Read the model definition and answer for the solid it produces. Units are mm, in the model's axes. Face numbers are marked on the shaded views. A direction names the side the tool comes from. Give positions to 0.01 mm unless a question says otherwise; leave off trailing zeros. Write each loop counter-clockwise with the first axis right and the second up, starting at its lowest first coordinate (ties: lowest second). Pieces come first, ordered by that corner, then holes. Notation, with made-up numbers: (-14.5, 25) -> (31.5, 25) arc R10 cw to (31.5, 42) -> close; hole circle Ø10 at (-33.75, 67.25). An arc over 180 degrees is marked (long way). Use a Markdown table: item, result.
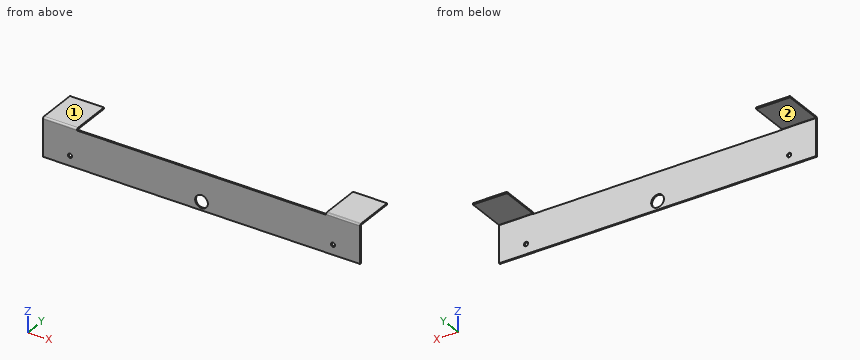
from build123d import *

# Parameters (mm, degrees)
SKETCH18_W                   = 711.2
SKETCH18_H                   = 3.175
BASE_FLANGE1_DEPTH           = 174.625
SKETCH23_W                   = 215.9
SKETCH23_H                   = 88.9
CUT_EXTRUDE1_DEPTH           = 630.633777431
SKETCH24_W                   = 127
SKETCH24_H                   = 34.925
CUT_EXTRUDE2_DEPTH           = 630.633777431
SKETCH25_W                   = 215.9
SKETCH25_H                   = 88.9
CUT_EXTRUDE3_DEPTH           = 630.633777431
SKETCH32_W                   = 558.8
SKETCH32_H                   = 92.075
CUT_EXTRUDE6_DEPTH           = 630.633777431
SKETCHED_START               = -106.274614162
SKETCHED_BEND1_OUTLINE_W     = 3.175
SKETCHED_BEND1_OUTLINE_H     = 88.9
SKETCHED_BEND1_OUTLINE_H_2   = 82.55
SKETCHED_BEND1_DEPTH         = 635
SKETCHED_START_2             = 528.725385838
SKETCHED_BEND1_2_DEPTH       = 76.2
SKETCHED_BEND1_3_OUTLINE_W   = 82.55
SKETCHED_BEND1_3_OUTLINE_H   = 3.175
SKETCHED_BEND1_3_DEPTH       = 711.2
SKETCHED_BEND1_4_OUTLINE_W   = 0.997512257
SKETCHED_BEND1_4_OUTLINE_H   = 3.175
SKETCHED_BEND1_4_OUTLINE_W_2 = 87.902487743
SKETCHED_BEND1_4_DEPTH       = 76.2
SKETCHED_BEND1_5_DEPTH       = 76.2
SKETCHED_BEND2_DEPTH         = 711.2
SKETCHED_BEND2_2_OUTLINE_W   = 3.175
SKETCHED_BEND2_2_OUTLINE_H   = 82.55
SKETCHED_BEND2_2_DEPTH       = 711.2
SKETCHED_BEND2_3_DEPTH       = 76.2
SKETCHED_BEND2_4_DEPTH       = 76.2
SKETCH35_R                   = 14.2875
SKETCH35_R_2                 = 4.7625
CUT_EXTRUDE7_DEPTH           = 619.781329454


# Read off the part's stored shape, not the designer's step: Sketched Bend1, Sketched Bend2
# Sheet-metal steps are written as plain solids
with BuildPart() as part:
    # Sketch18 → Base-Flange1 (new body)
    with BuildSketch(Plane.XY):
        with Locations((249.325385838, -1.5875)):
            Rectangle(SKETCH18_W, SKETCH18_H)
    extrude(amount=BASE_FLANGE1_DEPTH)

    # Sketch23 → Cut-Extrude1 (cut, through all)
    with BuildSketch(Plane(origin=(0, 0, 0), x_dir=(1, 0, 0), z_dir=(0, 1, 0))):
        with Locations((77.875385838, -44.45)):
            Rectangle(SKETCH23_W, SKETCH23_H)
    extrude(amount=-CUT_EXTRUDE1_DEPTH, mode=Mode.SUBTRACT)

    # Sketch24 → Cut-Extrude2 (cut, through all)
    with BuildSketch(Plane(origin=(0, 0, 0), x_dir=(1, 0, 0), z_dir=(0, 1, 0))):
        with Locations((249.325385838, -17.4625)):
            Rectangle(SKETCH24_W, SKETCH24_H)
    extrude(amount=-CUT_EXTRUDE2_DEPTH, mode=Mode.SUBTRACT)

    # Sketch25 → Cut-Extrude3 (cut, through all)
    with BuildSketch(Plane(origin=(0, 0, 0), x_dir=(1, 0, 0), z_dir=(0, 1, 0))):
        with Locations((420.775385838, -44.45)):
            Rectangle(SKETCH25_W, SKETCH25_H)
    extrude(amount=-CUT_EXTRUDE3_DEPTH, mode=Mode.SUBTRACT)

    # Sketch32 → Cut-Extrude6 (cut, through all)
    with BuildSketch(Plane.XZ.offset(3.175)):
        with Locations((249.325385838, 46.0375)):
            Rectangle(SKETCH32_W, SKETCH32_H)
    extrude(amount=-CUT_EXTRUDE6_DEPTH, mode=Mode.SUBTRACT)

    # Sketched Bend1 outline → Sketched Bend1 (cut)
    with BuildSketch(Plane.YZ.offset(SKETCHED_START)):
        with Locations((-1.5875, 44.45)):
            Rectangle(SKETCHED_BEND1_OUTLINE_W, SKETCHED_BEND1_OUTLINE_H)
        with Locations((-1.5875, 133.35)):
            Rectangle(SKETCHED_BEND1_OUTLINE_W, SKETCHED_BEND1_OUTLINE_H_2)
    extrude(amount=SKETCHED_BEND1_DEPTH, mode=Mode.SUBTRACT)

    # Sketched Bend1 2 outline → Sketched Bend1 2 (cut)
    with BuildSketch(Plane.YZ.offset(SKETCHED_START_2)):
        with BuildLine():
            ThreePointArc((-3.175, 92.005018799), (-0.896479843, 90.655319942), (0, 88.1634))
            Line((0, 88.1634), (0, 174.625))
            Line((0, 174.625), (-3.175, 174.625))
            Line((-3.175, 174.625), (-3.175, 92.005018799))
        make_face()
    extrude(amount=SKETCHED_BEND1_2_DEPTH, mode=Mode.SUBTRACT)



with BuildPart() as body_2:
    # Sketched Bend1 3 outline → Sketched Bend1 3 (new body)
    with BuildSketch(Plane.YZ.offset(SKETCHED_START)):
        with Locations((-45.447512257, 90.4875)):
            Rectangle(SKETCHED_BEND1_3_OUTLINE_W, SKETCHED_BEND1_3_OUTLINE_H)
    extrude(amount=SKETCHED_BEND1_3_DEPTH)


with BuildPart() as part_1:
    add(part.part)

    add(body_2.part)  # Sketched Bend1 4 merges body 2
    # Sketched Bend1 4 outline → Sketched Bend1 4 (add)
    with BuildSketch(Plane.YZ.offset(SKETCHED_START)):
        with Locations((-3.673756128, 90.4875)):
            Rectangle(SKETCHED_BEND1_4_OUTLINE_W, SKETCHED_BEND1_4_OUTLINE_H)
        with Locations((43.951243872, 90.4875)):
            Rectangle(SKETCHED_BEND1_4_OUTLINE_W_2, SKETCHED_BEND1_4_OUTLINE_H)
    extrude(amount=SKETCHED_BEND1_4_DEPTH)

    # Sketched Bend1 5 outline → Sketched Bend1 5 (add)
    with BuildSketch(Plane.YZ.offset(SKETCHED_START_2)):
        with BuildLine():
            Line((-4.172512257, 88.9), (-3.9116, 88.9))
            ThreePointArc((-3.9116, 88.9), (-3.390745145, 88.684254855), (-3.175, 88.1634))
            Line((-3.175, 88.1634), (-3.175, 92.005018799))
            ThreePointArc((-3.175, 92.005018799), (-3.541641581, 92.057465398), (-3.9116, 92.075))
            Line((-3.9116, 92.075), (-4.172512257, 92.075))
            Line((-4.172512257, 92.075), (-4.172512257, 88.9))
        make_face()
    extrude(amount=SKETCHED_BEND1_5_DEPTH)

    # Sketched Bend2 outline → Sketched Bend2 (cut)
    with BuildSketch(Plane.YZ.offset(SKETCHED_START)):
        with BuildLine():
            ThreePointArc((-4.102531056, 88.9), (-2.752832199, 91.178520157), (-0.260912257, 92.075))
            Line((-0.260912257, 92.075), (-86.722512257, 92.075))
            Line((-86.722512257, 92.075), (-86.722512257, 88.9))
            Line((-86.722512257, 88.9), (-4.102531056, 88.9))
        make_face()
        with BuildLine():
            Line((-0.997512257, 5.352487743), (-3.175, 5.352487743))
            Line((-3.175, 5.352487743), (-3.175, 0))
            Line((-3.175, 0), (0, 0))
            Line((0, 0), (0, 88.1634))
            ThreePointArc((0, 88.1634), (-0.017534602, 88.533358419), (-0.069981201, 88.9))
            Line((-0.069981201, 88.9), (-0.260912257, 88.9))
            ThreePointArc((-0.260912257, 88.9), (-0.781767112, 88.684254855), (-0.997512257, 88.1634))
            Line((-0.997512257, 88.1634), (-0.997512257, 5.352487743))
        make_face()
    extrude(amount=SKETCHED_BEND2_DEPTH, mode=Mode.SUBTRACT)

    # Sketched Bend2 2 outline → Sketched Bend2 2 (add)
    with BuildSketch(Plane.YZ.offset(SKETCHED_START)):
        with Locations((-2.585012257, 46.627487743)):
            Rectangle(SKETCHED_BEND2_2_OUTLINE_W, SKETCHED_BEND2_2_OUTLINE_H)
    extrude(amount=SKETCHED_BEND2_2_DEPTH)

    # Sketched Bend2 3 outline → Sketched Bend2 3 (add)
    with BuildSketch(Plane.YZ.offset(SKETCHED_START_2)):
        with BuildLine():
            ThreePointArc((-4.102531056, 88.9), (-4.154977655, 88.533358419), (-4.172512257, 88.1634))
            Line((-4.172512257, 88.1634), (-4.172512257, 87.902487743))
            Line((-4.172512257, 87.902487743), (-3.175, 87.902487743))
            Line((-3.175, 87.902487743), (-3.175, 88.1634))
            ThreePointArc((-3.175, 88.1634), (-3.390745145, 88.684254855), (-3.9116, 88.9))
            Line((-3.9116, 88.9), (-4.102531056, 88.9))
        make_face()
        with BuildLine():
            ThreePointArc((-0.260912257, 92.075), (-1.201151194, 91.960315235), (-2.086256128, 91.622985858))
            ThreePointArc((-2.086256128, 91.622985858), (-0.767990693, 90.491131747), (-0.069981201, 88.9))
            Line((-0.069981201, 88.9), (87.902487743, 88.9))
            Line((87.902487743, 88.9), (87.902487743, 92.075))
            Line((87.902487743, 92.075), (-0.260912257, 92.075))
        make_face()
    extrude(amount=SKETCHED_BEND2_3_DEPTH)

    # Sketched Bend2 4 outline → Sketched Bend2 4 (add)
    with BuildSketch(Plane.YZ.offset(SKETCHED_START)):
        with BuildLine():
            ThreePointArc((-4.102531056, 88.9), (-4.154977655, 88.533358419), (-4.172512257, 88.1634))
            Line((-4.172512257, 88.1634), (-4.172512257, 87.902487743))
            Line((-4.172512257, 87.902487743), (-0.997512257, 87.902487743))
            Line((-0.997512257, 87.902487743), (-0.997512257, 88.1634))
            ThreePointArc((-0.997512257, 88.1634), (-0.781767112, 88.684254855), (-0.260912257, 88.9))
            Line((-0.260912257, 88.9), (-4.102531056, 88.9))
        make_face()
    extrude(amount=SKETCHED_BEND2_4_DEPTH)

    # Sketch35 → Cut-Extrude7 (cut, through all)
    with BuildSketch(Plane(origin=(0, -4.172512257, 0), x_dir=(-1, 0, 0), z_dir=(0, -1, 0))):
        with Locations(Location((-249.325385838, -24.402487743, 0), (0, 0, 90))):
            Circle(SKETCH35_R)
        with Locations(Location((-544.399725838, -27.577487743, 0), (0, 0, 90))):
            Circle(SKETCH35_R_2)
        with Locations(Location((45.748954162, -27.577487743, 0), (0, 0, 90))):
            Circle(SKETCH35_R_2)
    extrude(amount=-CUT_EXTRUDE7_DEPTH, mode=Mode.SUBTRACT)


solid = part_1.part
Item 1: Each of these flat-tipped pins is pushed along its axis until it touches: P1, Ø25, axis at x = 109, z = 49.5, coming from the +Y side; P2, Ø2.5, axis at x = 258, y = -2.5, coming from the +Z side; P3, Ø17, axis at x = 249.33, z = 24.4, coming from the -Y side. Where does it stop, or does it pass through?
Return value:
| item | result |
|---|---|
| P1 | y = -1 |
| P2 | z = 87.9 |
| P3 | through |
Item 2: A tool of negligible diameter and unlimited length cuts with its end or side. For the marked faces 1 and 2, from which of +Z, -Z, +X, -X, +Y, -Y can it reach the whole face along a straight path? Write none if from no direction.
Return value:
| item | result |
|---|---|
| face 1 | +Z, +X, -X, +Y, -Y |
| face 2 | -Z, +X, -X, +Y |
Item 3: A cutting plane is placed at A-A (y = 77). Give the vertices of the cut face in (x, z) (3 decimals), then the cut area to 3 significant figures.
Return value:
| item | result |
|---|---|
| outline | (-106.275, 88.9) -> (-30.075, 88.9) -> (-30.075, 92.075) -> (-106.275, 92.075) -> close; (528.725, 88.9) -> (604.925, 88.9) -> (604.925, 92.075) -> (528.725, 92.075) -> close |
| area | 484 mm^2 |
Item 4: A cutting plane is placed at B-B (x = 196). Give the vertices of the cut face in (y, z), then the cut area to 3 significant figures.
Return value:
| item | result |
|---|---|
| outline | (-4.17, 5.35) -> (-1, 5.35) -> (-1, 87.9) -> (-4.17, 87.9) -> close |
| area | 262 mm^2 |
Item 5: A straight line is drawn through the part: line 1 along Y through (x, z) = (529, 61). Find the intervals that lie inside material, in ascending order. Write a range as [from, to].
Return value:
| item | result |
|---|---|
| line 1 | [-4.17, -1] |
